Autodesk Inventor part; units mm, degrees
ref_plane "YZ Plane" through (0, 0, 0) normal (1, 0, 0) x (0, 1, 0)
ref_plane "XZ Plane" through (0, 0, 0) normal (0, 1, 0) x (-1, 0, 0)
ref_plane "XY Plane" through (0, 0, 0) normal (0, 0, 1) x (1, 0, 0)
sketch "Esboço1" plane through (0, 0, 0) normal (0, 0, 1) x (1, 0, 0)
  line L0 (-28, 0) -> (28, 0) construction
  line L1 (0, -35) -> (0, 35) construction
  line L2 (-20, 25) -> (20, 25)
  line L3 (20, 25) -> (20, -25)
  line L4 (20, -25) -> (-20, -25)
  line L5 (-20, -25) -> (-20, 25)
  line L6 (-10, 25) -> (-10, -25) construction
  line L7 (10, 25) -> (10, -25) construction
  line L8 (-20, -10) -> (20, -10) construction
  point P0 (0, 0)
  point P1 (-10, -10)
  point P2 (10, -10)
  point P3 (0, -17.5)
  point P4 (0, 0)
  point P5 (0, 17.5)
  dimension "d0" = 40
  dimension "d1" = 50
  dimension "d2" = 20
  dimension "d3" = 15
  dimension "d13" = 35
extrude "Extrusão1" add sketch "Esboço1" against normal blind 25
hole "Furo1" at (-10, -10, 0) at (10, -10, 0) direction (0, 0, -1) diameter 6.5 end through all counterbore diameter 11 counterbore depth 10
hole "Furo2" at (0, -17.5, 0) at (0, 0, 0) at (0, 17.5, 0) direction (0, 0, -1) diameter 3.242 depth 15 tip angle 118
chamfer "Chanfro1" distance 1 angle 45 4 edges at (-20, -25, -12.5) (-20, 25, -12.5) (20, 25, -12.5) (20, -25, -12.5)
properties part number "Chapa Suporte Trilho 1" material "Poliacetal WT"
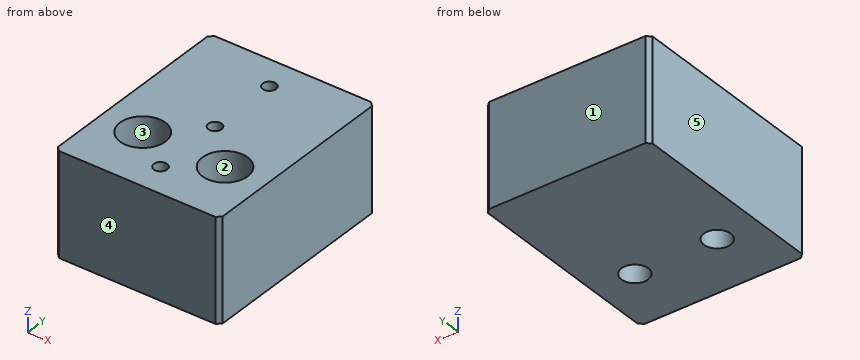
The listing builds one solid part. Answer for the finished solid, in the listing's coordinates (mm). Face numbers are marked on the shaded views. A direction names the side the tool comes from. Coordinates: 2 decimals unless noted, no trailing zeros. Order: outer loops, then holes, each group sorted by start corner. A loop starts at its lowest first (then second) coordinate and runs counter-clockwise, first axis right, second up. Notation, with made-up numbers: (30, 55) -> (42, 55) arc R23 ccw to (42, 79) -> close; hole circle Ø4 at (-19, 66). An arc over 180 degrees is marked (long way). Answer in a Markdown table with one row per item. Add a question column.
Item 1: Which of the six approach directions +Z, -Z, +X, -X, +Y, -Y give full straight-line access (tool end or side, diameter ignored) to the marked faces 1 and 2?
Item 2: Each of these flat-tipped pins is pushed along its axis until it touches: P1, Ø14.5, axis at x = 10, y = -10, coming from the +Z side; P2, Ø3, axis at x = 0, y = -17.5, coming from the +Z side; P3, Ø2.5, axis at x = 0, y = 17.5, coming from the +Z side; P4, Ø7.5, axis at x = 10, y = -10, coming from the +Z side. Where does it stop, or does it pass through?
Item 3: Find section D-D (z = -20.5). Write down the section's boundary in (x, y), then the cut area to 3 significant figures.
Item 4: Find section B-B (z = -2.25). Write down the section's boundary in (x, y).
Item 5: Find section A-A (x = -10). Write down the section's boundary in (y, z).
Item 6: Find the intervals of material crossed by L1, parallel to X at y = -10, z = -7; L2, parallel to Y at x = 10, z = -4.5; L3, parallel to X at y = -10, z = -14.75, in increasing order. Write a range as from..to.
Item 7: Determine the mould class of the marked faces 3, 4 and 5 for opening direction Y: +Y half, -Y half, draft (parallel to the pull), parting line (faces both ways), or undercut.
Item 8: Find section C-C (y = -10). Write down the section's boundary in (x, z).
Result set:
| question | item | result |
|---|---|---|
| 1 | face 1 | +Z, -Z, +X, -X, +Y |
| 1 | face 2 | +Z |
| 2 | P1 | stops at z = 0 |
| 2 | P2 | stops at z = -15.07 |
| 2 | P3 | stops at z = -15.22 |
| 2 | P4 | stops at z = -10 |
| 3 | outline | (-20, -24) -> (-19, -25) -> (19, -25) -> (20, -24) -> (20, 24) -> (19, 25) -> (-19, 25) -> (-20, 24) -> close; hole circle Ø6.5 at (-10, -10); hole circle Ø6.5 at (10, -10) |
| 3 | area | 1,930 mm² |
| 4 | outline | (-20, -24) -> (-19, -25) -> (19, -25) -> (20, -24) -> (20, 24) -> (19, 25) -> (-19, 25) -> (-20, 24) -> close; hole circle Ø11 at (-10, -10); hole circle Ø3.24 at (0, -17.5); hole circle Ø3.24 at (0, 0); hole circle Ø3.24 at (0, 17.5); hole circle Ø11 at (10, -10) |
| 5 | outline | (-25, -25) -> (-13.25, -25) -> (-13.25, -10) -> (-15.5, -10) -> (-15.5, 0) -> (-25, 0) -> close; (-6.75, -25) -> (25, -25) -> (25, 0) -> (-4.5, 0) -> (-4.5, -10) -> (-6.75, -10) -> close |
| 6 | L1 | x = -20..-15.5, -4.5..4.5, 15.5..20 |
| 6 | L2 | y = -25..-15.5, -4.5..25 |
| 6 | L3 | x = -20..-13.25, -6.75..6.75, 13.25..20 |
| 7 | face 3 | undercut |
| 7 | face 4 | -Y half |
| 7 | face 5 | draft |
| 8 | outline | (-20, -25) -> (-13.25, -25) -> (-13.25, -10) -> (-15.5, -10) -> (-15.5, 0) -> (-20, 0) -> close; (-6.75, -25) -> (6.75, -25) -> (6.75, -10) -> (4.5, -10) -> (4.5, 0) -> (-4.5, 0) -> (-4.5, -10) -> (-6.75, -10) -> close; (13.25, -25) -> (20, -25) -> (20, 0) -> (15.5, 0) -> (15.5, -10) -> (13.25, -10) -> close |
